```python
from build123d import *

# Parameters (mm, degrees)
SKETCH1_W           = 609.6
SKETCH1_H           = 609.6
SKETCH1_W_2         = 38.1
SKETCH1_H_2         = 127
BOSS_EXTRUDE1_DEPTH = 3.175


with BuildPart() as part:
    # Sketch1 → Boss-Extrude1 (new body)
    with BuildSketch(Plane(origin=(0, 0, 0), x_dir=(1, 0, 0), z_dir=(0, 1, 0))):
        Rectangle(SKETCH1_W, SKETCH1_H)
        Polygon((120.408154002, 135.779180095), (120.408154002, 262.779180095), (247.408154002, 262.779180095), (247.408154002, 224.679180095), (158.508154002, 224.679180095), (158.508154002, 135.779180095), align=None, mode=Mode.SUBTRACT)
        with Locations((0, 199.279180095)):
            Rectangle(SKETCH1_W_2, SKETCH1_H_2, mode=Mode.SUBTRACT)
        Polygon((-158.508154002, 224.679180095), (-158.508154002, 135.779180095), (-120.408154002, 135.779180095), (-120.408154002, 262.779180095), (-247.408154002, 262.779180095), (-247.408154002, 224.679180095), align=None, mode=Mode.SUBTRACT)
        Polygon((158.508154002, -224.679180095), (158.508154002, -135.779180095), (120.408154002, -135.779180095), (120.408154002, -262.779180095), (247.408154002, -262.779180095), (247.408154002, -224.679180095), align=None, mode=Mode.SUBTRACT)
        with Locations((0, -199.279180095)):
            Rectangle(SKETCH1_W_2, SKETCH1_H_2, mode=Mode.SUBTRACT)
        Polygon((-247.408154002, -224.679180095), (-158.508154002, -224.679180095), (-158.508154002, -135.779180095), (-120.408154002, -135.779180095), (-120.408154002, -262.779180095), (-247.408154002, -262.779180095), align=None, mode=Mode.SUBTRACT)
        with BuildLine():
            ThreePointArc((52.551332081, -135.779180095), (65.092340177, -148.636206032), (77.949366114, -136.095197937))
            add(Edge.make_bspline(
                [(77.949366114, -136.095197937), (77.962871775, -135.00976167), (78.051522279, -132.819994322), (78.461018982, -128.610747096), (79.391750695, -123.529893605), (81.140586923, -117.702146239), (84.288273438, -110.22828937), (89.724874356, -101.398698485), (98.52001314, -91.730852125), (109.296478393, -83.291620152), (125.7100411, -74.097744104), (144.107538407, -68.589807628), (162.008327299, -67.396780618), (174.562605493, -68.637977939), (185.730202076, -71.902172234), (195.230771881, -77.014054641), (201.820897642, -82.819870924), (206.398964756, -88.654208165), (209.481301131, -93.743351916), (212.177363153, -99.667795966), (214.042508359, -105.400408521), (215.255816836, -110.514072692), (216.01193439, -114.620965061), (216.502025281, -118.283361589), (216.801657973, -121.346084505), (216.920978677, -122.947020667), (216.971104363, -123.739711144)],
                knots=[0, 0, 0, 0, 0.015625, 0.03125, 0.0625, 0.09375, 0.125, 0.1875, 0.25, 0.3125, 0.375, 0.5, 0.5625, 0.625, 0.6875, 0.75, 0.8125, 0.84375, 0.875, 0.90625, 0.9375, 0.953125, 0.96875, 0.984375, 0.9921875, 1, 1, 1, 1], degree=3))
            ThreePointArc((216.971104363, -123.739711144), (230.447270979, -135.612913465), (242.3204733, -122.136746849))
            add(Edge.make_bspline(
                [(52.551332081, -135.779180095), (53.803993226, -35.104071896), (234.278707736, 5.036193149), (242.3204733, -122.136746849)],
                knots=[0, 0, 0, 0, 1, 1, 1, 1], degree=3))
        make_face(mode=Mode.SUBTRACT)
        with BuildLine():
            ThreePointArc((-52.551332081, 135.779180095), (-65.092340177, 148.636206032), (-77.949366114, 136.095197937))
            add(Edge.make_bspline(
                [(-77.949366114, 136.095197937), (-77.962871775, 135.00976167), (-78.051522279, 132.819994322), (-78.461018982, 128.610747096), (-79.391750695, 123.529893605), (-81.140586923, 117.702146239), (-84.288273438, 110.22828937), (-89.724874356, 101.398698485), (-98.52001314, 91.730852125), (-109.296478393, 83.291620152), (-125.7100411, 74.097744104), (-144.107538407, 68.589807628), (-162.008327299, 67.396780618), (-174.562605493, 68.637977939), (-185.730202076, 71.902172234), (-195.230771881, 77.014054641), (-201.820897642, 82.819870924), (-206.398964756, 88.654208165), (-209.481301131, 93.743351916), (-212.177363153, 99.667795966), (-214.042508359, 105.400408521), (-215.255816836, 110.514072692), (-216.01193439, 114.620965061), (-216.502025281, 118.283361589), (-216.801657973, 121.346084505), (-216.920978677, 122.947020667), (-216.971104363, 123.739711144)],
                knots=[0, 0, 0, 0, 0.015625, 0.03125, 0.0625, 0.09375, 0.125, 0.1875, 0.25, 0.3125, 0.375, 0.5, 0.5625, 0.625, 0.6875, 0.75, 0.8125, 0.84375, 0.875, 0.90625, 0.9375, 0.953125, 0.96875, 0.984375, 0.9921875, 1, 1, 1, 1], degree=3))
            ThreePointArc((-216.971104363, 123.739711144), (-230.447270979, 135.612913465), (-242.3204733, 122.136746849))
            add(Edge.make_bspline(
                [(-52.551332081, 135.779180095), (-53.803993226, 35.104071896), (-234.278707736, -5.036193149), (-242.3204733, 122.136746849)],
                knots=[0, 0, 0, 0, 1, 1, 1, 1], degree=3))
        make_face(mode=Mode.SUBTRACT)
        with BuildLine():
            ThreePointArc((-238.361805519, -109.276089344), (-227.793814923, -123.798402341), (-213.271501927, -113.230411744))
            add(Edge.make_bspline(
                [(-213.271501927, -113.230411744), (-213.151711371, -112.470336791), (-212.901399378, -110.942133808), (-212.376470719, -107.967853935), (-211.667401285, -104.350251745), (-210.737688056, -100.183113029), (-209.396326232, -94.848652891), (-207.537338772, -88.590365879), (-205.039618896, -81.703545889), (-202.297676371, -75.403179873), (-198.340291718, -67.72877181), (-192.86473475, -59.383344605), (-185.469393079, -50.978746481), (-177.159554076, -43.839947193), (-167.799053029, -37.731600761), (-153.784222926, -30.792133533), (-133.28509315, -24.22852654), (-104.453100091, -19.330230382), (-72.38586379, -16.682179087), (-38.055823436, -15.267140213), (-2.333026847, -13.913947785), (34.024700143, -11.346923243), (70.348040016, -6.174035434), (105.983184152, 3.16701171), (134.39986785, 15.91619513), (155.642723734, 29.956085882), (170.580590208, 42.556344707), (184.278786849, 57.320430485), (194.478117069, 71.453337622), (201.830548984, 83.861665804), (206.927792683, 93.718040184), (210.822379773, 102.401329596), (213.7158707, 109.613690679), (215.099625409, 113.341406131), (215.763927247, 115.202976942)],
                knots=[0, 0, 0, 0, 0.00390625, 0.0078125, 0.015625, 0.0234375, 0.03125, 0.046875, 0.0625, 0.078125, 0.09375, 0.125, 0.15625, 0.1875, 0.21875, 0.25, 0.3125, 0.375, 0.4375, 0.5, 0.5625, 0.625, 0.6875, 0.75, 0.8125, 0.84375, 0.875, 0.90625, 0.9375, 0.953125, 0.96875, 0.984375, 0.9921875, 1, 1, 1, 1], degree=3))
            ThreePointArc((215.763927247, 115.202976942), (208.071063547, 131.432574845), (191.841465644, 123.739711144))
            add(Edge.make_bspline(
                [(-238.361805519, -109.276089344), (-231.837247772, -67.877559295), (-143.94762142, 74.845593782), (129.599293897, -50.681317832), (191.841465644, 123.739711144)],
                knots=[0, 0, 0, 0, 0.18643952, 1, 1, 1, 1], degree=3))
        make_face(mode=Mode.SUBTRACT)
    extrude(amount=BOSS_EXTRUDE1_DEPTH)


solid = part.part
```
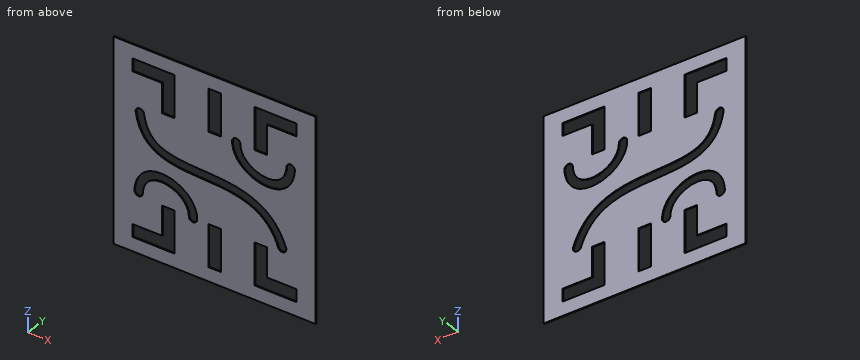
Source: CAD feature listing. Evaluate the final solid. Frame: model axes, mm. Give positions to 0.01 mm unless a question says otherwise; leave off trailing zeros. Write each loop counter-clockwise with the first axis right and the second up, starting at its lowest first coordinate (ties: lowest second). Pieces come first, ordered by that corner, then holes.
1. Section query B-B (z = -215.5). Return the cut outline in (x, y) (3 decimals).
2. Material intervals for line 1 along X through (y, z) = (2.05, -230.5); line 2 along X through (y, z) = (2, -207.5); line 3 along Z through (x, y) = (223, 1.65), sorted ascending.
3. Section query C-C (x = 149). Count the separate pieces of the cut face and the enclosed holes in it, then the cut area to 3 significant figures.
4. Section query A-A (z = 242.5). Return the cut outline in (x, y) (3 decimals), then the cut area to 3 significant figures.
Output values:
1. outline: (-304.8, 0) - (-158.508, 0) - (-158.508, 3.175) - (-304.8, 3.175) - close; (-120.408, 0) - (-19.05, 0) - (-19.05, 3.175) - (-120.408, 3.175) - close; (19.05, 0) - (120.408, 0) - (120.408, 3.175) - (19.05, 3.175) - close; (158.508, 0) - (304.8, 0) - (304.8, 3.175) - (158.508, 3.175) - close
2. line 1: x = -304.8 to -247.41, -120.41 to -19.05, 19.05 to 120.41, 247.41 to 304.8
2. line 2: x = -304.8 to -158.51, -120.41 to -19.05, 19.05 to 120.41, 158.51 to 304.8
2. line 3: z = -304.8 to -262.78, -224.68 to 68.78, 133.76 to 224.68, 262.78 to 304.8
3. separate pieces: 5
3. enclosed holes: 0
3. area: 946 mm2
4. outline: (-304.8, 0) - (-247.408, 0) - (-247.408, 3.175) - (-304.8, 3.175) - close; (-120.408, 0) - (-19.05, 0) - (-19.05, 3.175) - (-120.408, 3.175) - close; (19.05, 0) - (120.408, 0) - (120.408, 3.175) - (19.05, 3.175) - close; (247.408, 0) - (304.8, 0) - (304.8, 3.175) - (247.408, 3.175) - close
4. area: 1,010 mm2
